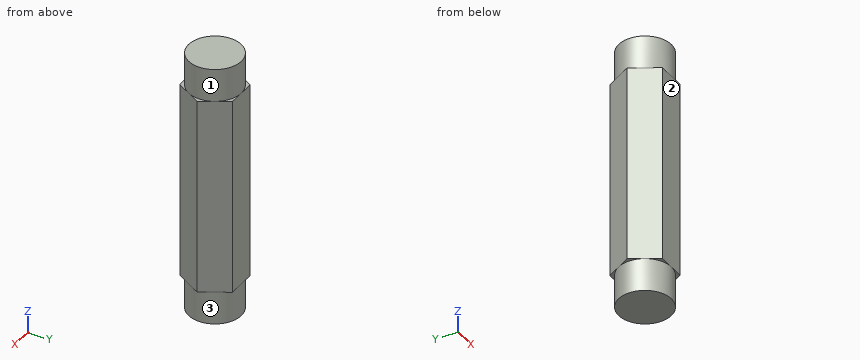
from build123d import *

# Parameters (mm, degrees)
BOSS_EXTRUDE1_DEPTH     = 31.75
SKETCH2_R               = 8.89
SKETCH2_R_2             = 6.35
CUT_EXTRUDE_THIN1_DEPTH = 7.9375


with BuildPart() as part:
    # Sketch1 → Boss-Extrude1 (new, symmetric)
    with BuildSketch(Plane.XY):
        Polygon((7.332348419, 0), (3.666174209, 6.35), (-3.666174209, 6.35), (-7.332348419, 0), (-3.666174209, -6.35), (3.666174209, -6.35), align=None)
    extrude(amount=BOSS_EXTRUDE1_DEPTH, both=True)

    # Sketch2 → Cut-Extrude-Thin1 (cut)
    with BuildSketch(Plane.XY.offset(31.75)):
        Circle(SKETCH2_R)
        Circle(SKETCH2_R_2, mode=Mode.SUBTRACT)
    cut_extrude_thin1 = extrude(amount=-CUT_EXTRUDE_THIN1_DEPTH, mode=Mode.SUBTRACT)

    # Mirror1: Cut-Extrude-Thin1 across plane
    add(cut_extrude_thin1.mirror(Plane.XY), mode=Mode.SUBTRACT)


solid = part.part
Verification items for the finished model (mm, model axes). Face numbers are marked on the shaded views. A direction names the side the tool comes from. Give positions to 0.01 mm unless a question says otherwise; leave off trailing zeros. Write each loop counter-clockwise with the first axis right and the second up, starting at its lowest first coordinate (ties: lowest second). Pieces come first, ordered by that corner, then holes. Notation, with made-up numbers: M 45,65 L 73,65 A30 cw 73,91 Z; hole C 69,38 d8. An arc over 180 degrees is marked long. Write item = value, one per line.
(1) Material ranges on line 1 (Z direction, x = -4, y = 5.5); line 2 (X direction, y = -0.25, z = 27.5); line 3 (X direction, y = -4.75, z = 5.5), recorded low to high.
Found:
line_1 = -23.81 to 23.81
line_2 = -6.35 to 6.35
line_3 = -4.59 to 4.59
(2) Access from +Z, -Z, +X, -X, +Y, -Y to the whole of each face (thin tool, end or side, straight path). Record for the marked faces 1, 2 and 3.
Found:
face_1 = +Z
face_2 = +Z, -Z, +X, -X, -Y
face_3 = -Z
(3) Sectioned sample at A-A (z = -3). Record the cut outline in (x, y), then the cut area to 3 significant figures.
Found:
outline = M -7.33,0 L -3.67,-6.35 L 3.67,-6.35 L 7.33,0 L 3.67,6.35 L -3.67,6.35 Z
area = 140 mm2
(4) Sectioned sample at B-B (x = 4.25). Record the cut outline in (y, z).
Found:
outline = M -5.34,-23.81 L -4.72,-23.81 L -4.72,-31.75 L 4.72,-31.75 L 4.72,-23.81 L 5.34,-23.81 L 5.34,23.81 L 4.72,23.81 L 4.72,31.75 L -4.72,31.75 L -4.72,23.81 L -5.34,23.81 Z
(5) Go/stop test with flat-tipped pins: pin 1 Ø2 at (y, z) = (-5, 14.5) entering from +X; pin 2 Ø6 at (y, z) = (-4.5, -10.5) entering from +X; pin 3 Ø2 at (x, y) = (6.5, -0.5) entering from +Z. Record where each tip stops, or that it passes through.
Found:
pin_1 = 5.02
pin_2 = 6.47
pin_3 = 31.75
